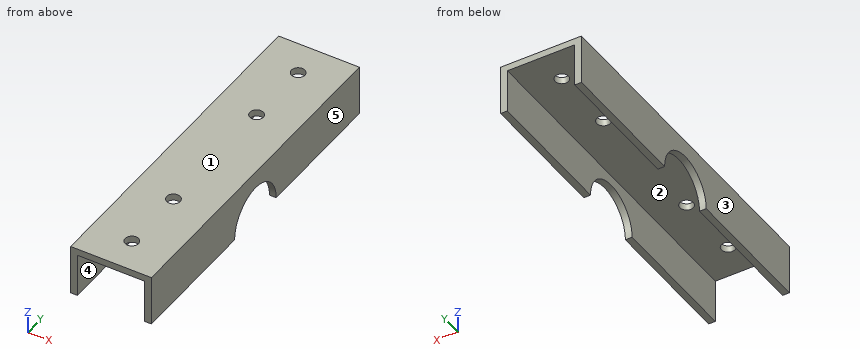
```python
from build123d import *

# Parameters (mm, degrees)
F1_DEPTH = 100
F2_R     = 10
F3_DEPTH = 25
F4_R     = 2
F5_DEPTH = 25


with BuildPart() as f1:
    # F0 (on Front) → F1 (new body)
    with BuildSketch(Plane.XZ):
        Polygon((0, -15), (0, 0), (-24, 0), (-24, -15), (-22, -15), (-22, -2), (-2, -2), (-2, -15), align=None)
    extrude(amount=F1_DEPTH)

    # F2 (on face) → F3 (cut)
    with BuildSketch(Plane.YZ):
        with Locations((-50, -15)):
            Circle(F2_R)
    extrude(amount=-F3_DEPTH, mode=Mode.SUBTRACT)

    # F4 (on face) → F5 (cut)
    with BuildSketch(Plane.XY):
        with Locations((-12, -90)):
            Circle(F4_R)
        with Locations((-12, -70)):
            Circle(F4_R)
        with Locations((-12, -30)):
            Circle(F4_R)
        with Locations((-12, -10)):
            Circle(F4_R)
    extrude(amount=-F5_DEPTH, mode=Mode.SUBTRACT)


solid = f1.part
```
The listing builds one solid part. Answer for the finished solid, in the listing's coordinates (mm). Face numbers are marked on the shaded views. A direction names the side the tool comes from. Give positions to 0.01 mm unless a question says otherwise; leave off trailing zeros. Order: outer loops, then holes, each group sorted by start corner. A loop starts at its lowest first (then second) coordinate and runs counter-clockwise, first axis right, second up.
Item 1: For a pull along X with two mould halves and no side action, classify the marked faces 1, 2 and 3 as pulls with the +X half, pulls with the -X half, needs draft (parallel to the pull), parting line crosses it, or undercut.
From the geometry:
face 1: needs draft
face 2: undercut
face 3: pulls with the -X half
Item 2: The part is cut by section C-C, the plane y = -21.5. Give the vertices of the cut face in (x, z).
From the geometry:
outline: (-24, -15) - (-22, -15) - (-22, -2) - (-2, -2) - (-2, -15) - (0, -15) - (0, 0) - (-24, 0) - close
Item 3: Which of the six approach directions +Z, -Z, +X, -X, +Y, -Y give full straight-line access (tool end or side, diameter ignored) to the marked faces 4 and 5?
From the geometry:
face 4: -Z, +Y, -Y
face 5: +Z, -Z, +X, +Y, -Y
Item 4: Given pin 1 Ø4.5 at (x, y) = (-12, -10) entering from -Z, flat-ended and moving along its own axis, determine where the tip first touches the part or whether it passes through.
From the geometry:
pin 1: stops at z = -2
Item 5: The part is cut by section D-D, the plane x = -6.5. Give the vertices of the cut face in (y, z), and give its area (3 significant figures).
From the geometry:
outline: (-100, -2) - (0, -2) - (0, 0) - (-100, 0) - close
area: 200 mm2
Item 6: The part is cut by section A-A, the plane z = -11. Give the vertices of the cut face in (x, y).
From the geometry:
outline: (-24, -100) - (-22, -100) - (-22, -59.17) - (-24, -59.17) - close; (-24, -40.83) - (-22, -40.83) - (-22, 0) - (-24, 0) - close; (-2, -100) - (0, -100) - (0, -59.17) - (-2, -59.17) - close; (-2, -40.83) - (0, -40.83) - (0, 0) - (-2, 0) - close
Item 7: Find the intervals of material crossed by probe 1 along Y at (x, z) = (-12, -1.25); probe 2 along X at (y, z) = (-12.5, -6.25); probe 3 along Z at (x, y) = (-4.75, -66), in increasing order.
From the geometry:
probe 1: y = -100 to -92, -88 to -72, -68 to -32, -28 to -12, -8 to 0
probe 2: x = -24 to -22, -2 to 0
probe 3: z = -2 to 0
Item 8: The part is cut by section B-B, the plane y = -70. Give the vertices of the cut face in (x, z), and give its area (3 significant figures).
From the geometry:
outline: (-24, -15) - (-22, -15) - (-22, -2) - (-14, -2) - (-14, 0) - (-24, 0) - close; (-10, -2) - (-2, -2) - (-2, -15) - (0, -15) - (0, 0) - (-10, 0) - close
area: 92.0 mm2
